```python
from build123d import *

# Parameters (mm, degrees)
F0_W     = 147.747025
F0_H     = 70.374168
F1_DEPTH = 52.5
F2_R     = 23.006046
F3_DEPTH = 14.6
F5_DEPTH = 25


with BuildPart() as f1:
    # F0 (on Top) → F1 (new body)
    with BuildSketch(Plane.XY):
        with Locations((8.377738, -8.017082)):
            Rectangle(F0_W, F0_H)
    extrude(amount=F1_DEPTH)

    # F2 (on face) → F3 (cut)
    with BuildSketch(Plane.XY.offset(52.5)):
        with Locations((12.676676, -2.870056)):
            Circle(F2_R)
    extrude(amount=-F3_DEPTH, mode=Mode.SUBTRACT)

    # F4 (on face) → F5 (cut)
    with BuildSketch(Plane.XY.offset(37.9)):
        with BuildLine():
            Line((24.04391, 0), (3.486699, 0))
            ThreePointArc((3.486699, 0), (2.779592, -0.292893), (2.486699, -1))
            Line((2.486699, -1), (2.486699, -13.646441))
            ThreePointArc((2.486699, -13.646441), (2.779592, -14.353548), (3.486699, -14.646441))
            Line((3.486699, -14.646441), (24.04391, -14.646441))
            ThreePointArc((24.04391, -14.646441), (24.751016, -14.353548), (25.04391, -13.646441))
            Line((25.04391, -13.646441), (25.04391, -1))
            ThreePointArc((25.04391, -1), (24.751016, -0.292893), (24.04391, 0))
        make_face()
    extrude(amount=-F5_DEPTH, mode=Mode.SUBTRACT)


solid = f1.part
```
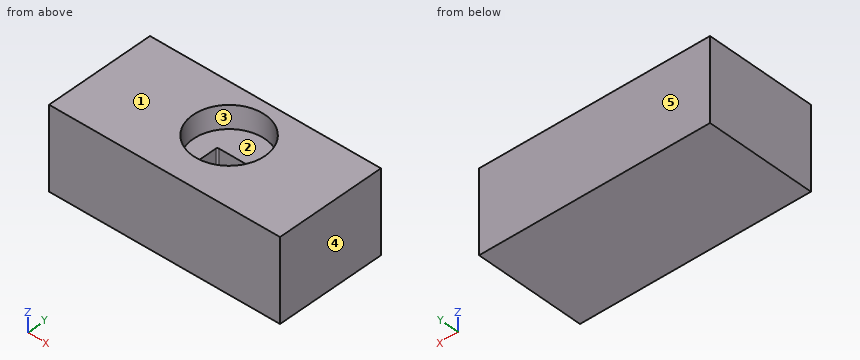
For this review, take the finished solid that the model builds, in its own axes (mm). Face numbers are marked on the shaded views. A direction names the side the tool comes from. Coordinates: 2 decimals unless noted, no trailing zeros. Write each loop counter-clockwise with the first axis right and the second up, starting at its lowest first coordinate (ties: lowest second). Pieces come first, ordered by that corner, then holes.
(1) Tool access review of the marked faces 1 and 2: name each direction out of +Z, -Z, +X, -X, +Y, -Y from which nothing blocks a thin tool from reaching the whole face with its end or side.
(2) Add section C-C on x = 12. Give the boundary of the cut face in (y, z), then the cut area to 3 significant figures.
(3) Add section D-D on y = -9. Give the boundary of the cut face in (x, z).
(4) The part is to be moulded in two halves that separate along X. For the marked faces 3, 4 and 5, say which applies: +X half, -X half, draft (parallel to the pull), parting line (faces both ways), or undercut.
(5) Wall thickness on probe 1 along Y at (x, z) = (23.5, 50); probe 2 along X at (y, z) = (12.5, 50); probe 3 along Z at (x, y) = (5.5, -0.5): over which ranges is each line inside the solid? List them lowest first.
(6) For pin 1 Ø4.5 at (x, y) = (16.5, -4) entering from +Z; pin 2 Ø4 at (x, y) = (28.5, 7) entering from -Z; pin 3 Ø14 at (x, y) = (17, -13.5) entering from +Z, all flat-tipped, find the tip position at first contact; note any pin that passes through.
(7) Add section A-A on z = 33.5. Give the boundary of the cut face in (x, y), then the cut area to 3 significant figures.
(8) Add section B-B on y = 3. Give the boundary of the cut face in (x, z), then the cut area to 3 significant figures.
Answer sheet:
1. face 1: +Z, +X, -X, +Y, -Y
1. face 2: +Z
2. outline: (-43.2, 0) - (27.17, 0) - (27.17, 52.5) - (20.13, 52.5) - (20.13, 37.9) - (0, 37.9) - (0, 12.9) - (-14.65, 12.9) - (-14.65, 37.9) - (-25.87, 37.9) - (-25.87, 52.5) - (-43.2, 52.5) - close
2. area: 2,660 mm2
3. outline: (-65.5, 0) - (82.25, 0) - (82.25, 52.5) - (34.85, 52.5) - (34.85, 37.9) - (25.04, 37.9) - (25.04, 12.9) - (2.49, 12.9) - (2.49, 37.9) - (-9.5, 37.9) - (-9.5, 52.5) - (-65.5, 52.5) - close
4. face 3: undercut
4. face 4: +X half
4. face 5: draft
5. probe 1: y = -43.2 to -23.17, 17.43 to 27.17
5. probe 2: x = -65.5 to -4.44, 29.8 to 82.25
5. probe 3: z = 0 to 12.9
6. pin 1: stops at z = 12.9
6. pin 2: stops at z = 0
6. pin 3: stops at z = 37.9
7. outline: (-65.5, -43.2) - (82.25, -43.2) - (82.25, 27.17) - (-65.5, 27.17) - close; hole (2.49, -13.65) arc R1 ccw to (3.49, -14.65) - (24.04, -14.65) arc R1 ccw to (25.04, -13.65) - (25.04, -1) arc R1 ccw to (24.04, 0) - (3.49, 0) arc R1 ccw to (2.49, -1) - close
7. area: 10,100 mm2
8. outline: (-65.5, 0) - (82.25, 0) - (82.25, 52.5) - (34.92, 52.5) - (34.92, 37.9) - (-9.57, 37.9) - (-9.57, 52.5) - (-65.5, 52.5) - close
8. area: 7,110 mm2
